Check sheet for the modelled part. Datum: model origin and axes. Units: mm. A direction names the side the tool comes from. Give positions to 0.01 mm unless a question says otherwise; leave off trailing zeros. Order: outer loops, then holes, each group sorted by start corner. A loop starts at its lowest first (then second) coordinate and runs counter-clockwise, first axis right, second up.
Item 1: Access from +Z, -Z, +X, -X, +Y, -Y to the whole of each face (thin tool, end or side, straight path). Record for faces 4 (the flat face through (19, 2, 0)), 5 (the flat face through (1, 0, 0)), 6 (the flat face through (-20, -9, 10)).
Item 2: Release check for a two-part mould opening along Y. For faces 1 (the flat face through (-20, -9, -6)), 2 (the cylindrical face through (-21.54, -13.07, 13.5)), 3 (the flat face through (-24, -5, 0)) record: released by +Y, released by -Y, zero draft, split by the parting line, or undercut.
Item 3: Material ranges on line 1 along Y through (x, z) = (-22.85, 8); line 2 along Y through (x, z) = (-19.3, 8); line 3 along X through (y, z) = (-12.25, -4.5), recorded low to high.
Item 4: Sectioned sample at C-C on y = -7. Record the boundary of the cut face in (x, z), and give its area (3 significant figures).
Item 5: Sectioned sample at A-A on y = 1.5. Record the boundary of the cut face in (x, z), and give its area (3 significant figures).
Item 6: Sectioned sample at D-D on z = 8. Record the boundary of the cut face in (x, y).
Item 7: Sectioned sample at B-B on z = 0. Record the boundary of the cut face in (x, y).
Item 8: Gauge pin test, flat ends, axial feed: P1, Ø6, axis at y = -7, z = -8, coming from the +X side; P2, Ø9, axis at x = 8, z = 6, coming from the -Y side; P3, Ø4, axis at y = -5, z = 0.5, coming from the +X side. Record the tip position at first contact, or that the pin passes through.
from build123d import *

# Parameters (mm, degrees)
SKETCH1_W           = 38
SKETCH1_H           = 30
BOSS_EXTRUDE1_DEPTH = 3.5
SKETCH2_W           = 30
SKETCH2_H           = 18
BOSS_EXTRUDE2_DEPTH = 5
SKETCH3_R           = 4
CUT_EXTRUDE1_DEPTH  = 1
SKETCH4_R           = 2.5
CUT_EXTRUDE2_DEPTH  = 5
SKETCH5_R           = 2.5
CUT_EXTRUDE3_DEPTH  = 5
FILLET1_R           = 10
FILLET2_R           = 2
FILLET3_R           = 5


with BuildPart() as part:
    # Sketch1 → Boss-Extrude1 (new body)
    with BuildSketch(Plane(origin=(0, 0, 0), x_dir=(1, 0, 0), z_dir=(0, 1, 0))):
        Rectangle(SKETCH1_W, SKETCH1_H)
    extrude(amount=BOSS_EXTRUDE1_DEPTH)

    # Sketch2 → Boss-Extrude2 (add)
    with BuildSketch(Plane.ZY.offset(19)):
        with Locations((0, -5.5)):
            Rectangle(SKETCH2_W, SKETCH2_H)
    extrude(amount=BOSS_EXTRUDE2_DEPTH)

    # Sketch3 → Cut-Extrude1 (cut)
    with BuildSketch(Plane(origin=(-19, 0, 0), x_dir=(0, 0, -1), z_dir=(1, 0, 0))):
        with Locations((-8, -7)):
            Circle(SKETCH3_R)
        with Locations((8, -7)):
            Circle(SKETCH3_R)
    extrude(amount=-CUT_EXTRUDE1_DEPTH, mode=Mode.SUBTRACT)

    # Sketch4 → Cut-Extrude2 (cut)
    with BuildSketch(Plane(origin=(-20, 0, 0), x_dir=(0, 0, -1), z_dir=(1, 0, 0))):
        with Locations((-8, -7)):
            Circle(SKETCH4_R)
        with Locations((8, -7)):
            Circle(SKETCH4_R)
    extrude(amount=-CUT_EXTRUDE2_DEPTH, mode=Mode.SUBTRACT)

    # Sketch5 → Cut-Extrude3 (cut)
    with BuildSketch(Plane(origin=(0, 3.5, 0), x_dir=(1, 0, 0), z_dir=(0, 1, 0))):
        with Locations((9.25, 0)):
            Circle(SKETCH5_R)
    extrude(amount=-CUT_EXTRUDE3_DEPTH, mode=Mode.SUBTRACT)

    # Fillet1
    fillet1_edges = [part.edges().sort_by_distance(p)[0] for p in [
        (19, 1.75, -15),
        (19, 1.75, 15),
    ]]
    fillet(fillet1_edges, radius=FILLET1_R)

    # Fillet2
    fillet2_edges = [part.edges().sort_by_distance(p)[0] for p in [
        (-19, 0, 0),
    ]]
    fillet(fillet2_edges, radius=FILLET2_R)

    # Fillet3
    fillet3_edges = [part.edges().sort_by_distance(p)[0] for p in [
        (-21.5, -14.5, -15),
        (-21.5, -14.5, 15),
    ]]
    fillet(fillet3_edges, radius=FILLET3_R)


solid = part.part
Report:
1. face 4: +Z, -Z, +X, +Y, -Y
1. face 5: +Z, -Z, +X, -Y
1. face 6: +X
2. face 1: undercut
2. face 2: released by -Y
2. face 3: zero draft
3. line 1: y = -14.5 to -9.5, -4.5 to 3.5
3. line 2: y = -14.5 to -11, -3 to 3.5
3. line 3: x = -24 to -19
4. outline: (-24, -15) - (-19, -15) - (-19, -12) - (-20, -12) - (-20, -10.5) - (-24, -10.5) - close; (-24, -5.5) - (-20, -5.5) - (-20, -4) - (-19, -4) - (-19, 4) - (-20, 4) - (-20, 5.5) - (-24, 5.5) - close; (-24, 10.5) - (-20, 10.5) - (-20, 12) - (-19, 12) - (-19, 15) - (-24, 15) - close
4. area: 94.0 mm2
5. outline: (-24, -15) - (9, -15) arc R10 ccw to (19, -5) - (19, 5) arc R10 ccw to (9, 15) - (-24, 15) - close; hole circle Ø5 at (9.25, 0)
5. area: 1,230 mm2
6. outline: (-24, -14.5) - (-19, -14.5) - (-19, -11) - (-20, -11) - (-20, -9.5) - (-24, -9.5) - close; (-24, -4.5) - (-20, -4.5) - (-20, -3) - (-19, -3) - (-19, -2) arc R2 cw to (-17, 0) - (18.54, 0) - (18.54, 3.5) - (-24, 3.5) - close
7. outline: (-24, -14.5) - (-19, -14.5) - (-19, -2) arc R2 cw to (-17, 0) - (6.75, 0) - (6.75, 3.5) - (-24, 3.5) - close; (11.75, 0) - (19, 0) - (19, 3.5) - (11.75, 3.5) - close
8. P1: stops at x = -20
8. P2: stops at y = 0
8. P3: stops at x = -19
